```python
from build123d import *

# Parameters (mm, degrees)
F1_DEPTH  = 10
F3_D      = 2
F3_DEPTH  = 12
F3_TIP    = 0.600860619
F4_R      = 1
F5_DEPTH  = 13
F7_DEPTH  = 25
F9_DEPTH  = 9.8022701892
F11_DEPTH = 12.5


with BuildPart() as f1:
    # F0 (on Front) → F1 (new body)
    with BuildSketch(Plane.XZ):
        with BuildLine():
            Line((-4.3301270189, 21.3675134595), (-20.6698729811, -6.9337567297))
            ThreePointArc((-20.6698729811, -6.9337567297), (-20.6698729811, -11.9337567297), (-16.3397459622, -14.4337567297))
            Line((-16.3397459622, -14.4337567297), (16.3397459622, -14.4337567297))
            ThreePointArc((16.3397459622, -14.4337567297), (20.6698729811, -11.9337567297), (20.6698729811, -6.9337567297))
            Line((20.6698729811, -6.9337567297), (4.3301270189, 21.3675134595))
            ThreePointArc((4.3301270189, 21.3675134595), (0, 23.8675134595), (-4.3301270189, 21.3675134595))
        make_face()
    extrude(amount=F1_DEPTH)

    # F3
    with Locations(Plane.XZ.offset(10)):
        with Locations((0, 18.8675134595), (0, 0), (16.3397459622, -9.4337567297), (-16.3397459622, -9.4337567297)):
            Hole(F3_D / 2, depth=F3_DEPTH)
            with Locations((0, 0, -(F3_DEPTH + F3_TIP / 2))):  # 118° drill point
                Cone(0, F3_D / 2, F3_TIP, mode=Mode.SUBTRACT)

    # F4 (on face) → F5 (join)
    with BuildSketch(Plane(origin=(0, 0, 0), x_dir=(-1, 0, 0), z_dir=(0, 1, 0))):
        with BuildLine():
            Line((-7, 5.5662432703), (-7, -14.4337567297))
            Line((-7, -14.4337567297), (16.3397459622, -14.4337567297))
            ThreePointArc((16.3397459622, -14.4337567297), (20.6698729811, -11.9337567297), (20.6698729811, -6.9337567297))
            Line((20.6698729811, -6.9337567297), (4.3301270189, 21.3675134595))
            ThreePointArc((4.3301270189, 21.3675134595), (0, 23.8675134595), (-4.3301270189, 21.3675134595))
            Line((-4.3301270189, 21.3675134595), (-13.4529946162, 5.5662432703))
            Line((-13.4529946162, 5.5662432703), (-7, 5.5662432703))
        make_face()
        with Locations((16.3397459622, -9.4337567297)):
            Circle(F4_R, mode=Mode.SUBTRACT)
        Circle(F4_R, mode=Mode.SUBTRACT)
        with Locations((0, 18.8675134595)):
            Circle(F4_R, mode=Mode.SUBTRACT)
        with Locations((16.3397459622, -9.4337567297)):
            Circle(F4_R)
        Circle(F4_R)
        with Locations((0, 18.8675134595)):
            Circle(F4_R)
    extrude(amount=F5_DEPTH)

    # F6 (on face) → F7 (join)
    with BuildSketch(Plane(origin=(0, 13, 0), x_dir=(-1, 0, 0), z_dir=(0, 1, 0))):
        with BuildLine():
            Line((8.5455173281, 14.0662432703), (4.3301270189, 21.3675134595))
            ThreePointArc((4.3301270189, 21.3675134595), (0, 23.8675134595), (-4.3301270189, 21.3675134595))
            Line((-4.3301270189, 21.3675134595), (-8.5455173281, 14.0662432703))
            Line((-8.5455173281, 14.0662432703), (8.5455173281, 14.0662432703))
        make_face()
    extrude(amount=F7_DEPTH)

    # F8 (on face) → F9 (cut, through all)
    with BuildSketch(Plane(origin=(0, 0, 14.0662432703), x_dir=(1, 0, 0), z_dir=(0, 0, -1))):
        with BuildLine():
            Line((-8.5455173281, -38), (-8.5455173281, -20.0741813354))
            ThreePointArc((-8.5455173281, -20.0741813354), (-24.827324347, -44.9686543445), (4.0910069124, -38))
            Line((4.0910069124, -38), (-8.5455173281, -38))
        make_face()
        with BuildLine():
            ThreePointArc((4.0910069124, -38), (4.2102022324, -36.8778052582), (4.25, -35.75))
            ThreePointArc((4.25, -35.75), (0.6449933996, -25.6324835743), (-8.5455173281, -20.0741813354))
            Line((-8.5455173281, -20.0741813354), (-8.5455173281, -38))
            Line((-8.5455173281, -38), (4.0910069124, -38))
        make_face()
    extrude(amount=-F9_DEPTH, mode=Mode.SUBTRACT)

    # F10 (on Right) → F11 (cut, symmetric)
    with BuildSketch(Plane.YZ):
        Polygon((13, 23.8675134595), (38, 14.0662432703), (39, 14.0662432703), (39, 24.8675134595), (13, 24.8675134595), align=None)
    extrude(amount=F11_DEPTH, both=True, mode=Mode.SUBTRACT)


solid = f1.part
```
Geometry check sheet. Reference: the model listing, model coordinates, mm. A direction names the side the tool comes from. Round coordinates to 2 decimals unless told otherwise and drop trailing zeros. Write each loop counter-clockwise with the first axis right and the second up, starting at its lowest first coordinate (ties: lowest second). Pieces come first, ordered by that corner, then holes. Notation, with made-up numbers: (-33.5, 60.25) -> (-27.5, 60.25) arc R30 cw to (-27.5, 86.25) -> close; hole circle Ø10 at (59.25, 80.5). An arc over 180 degrees is marked (long way). Put each result on its own line as item: value.
1) Depth check by flat-ended pin: P1, Ø3, axis at y = -1, z = -1, coming from the +X side; P2, Ø6, axis at x = 6.5, z = -0.5, coming from the +Y side; P3, Ø6.5, axis at y = 9.5, z = -2.5, coming from the +X side. Enter the tip coordinate at first touch or a pass-through.
Recorded:
P1: stops at x = 18.11
P2: stops at y = 13
P3: stops at x = 7
2) Cross-section at D-D, the plane y = 14. Enter the section's corners in (x, z).
Recorded:
outline: (-8.55, 14.07) -> (8.55, 14.07) -> (4.33, 21.37) arc R5 ccw to (1.94, 23.48) -> (-1.94, 23.48) arc R5 ccw to (-4.33, 21.37) -> close
3) Release check for a two-part mould opening along X. For faces 1 (the face through (-17.294, -4.93, -9.133)), 2 (the face through (-20.63, 1.34, -12)), 3 (the face through (10, 6, 5.566)), 4 (the face through (-0.073, 1.219, 23.867)) record: pulls with the +X half, pulls with the -X half, needs draft (parallel to the pull), parting line crosses it, or undercut.
Recorded:
face 1: undercut
face 2: pulls with the -X half
face 3: needs draft
face 4: parting line crosses it
4) Access from +Z, -Z, +X, -X, +Y, -Y to the whole of each face (thin tool, end or side, straight path). Record for faces 5 (the face through (0, -5, -1)), 6 (the face through (12, 0, -7)), 7 (the face through (0, -10, -4)), 8 (the face through (2, 23, 14.066)).
Recorded:
face 5: -Y
face 6: -Z, +X, +Y
face 7: +Z, -Z, +X, -X, -Y
face 8: -Z, +X, -X, +Y
5) Cross-section at B-B, the plane x = 0. Enter the section's corners in (y, z).
Recorded:
outline: (-10, -14.43) -> (13, -14.43) -> (13, 14.07) -> (24.89, 14.07) -> (24.89, 19.21) -> (13, 23.87) -> (-10, 23.87) -> (-10, 19.87) -> (0, 19.87) -> (0, 17.87) -> (-10, 17.87) -> (-10, 1) -> (0, 1) -> (0, -1) -> (-10, -1) -> close
6) Cross-section at A-A, the plane y = -2. Enter the section's corners in (x, z), plus the area to 3 significant figures.
Recorded:
outline: (-20.67, -6.93) arc R5 ccw to (-16.34, -14.43) -> (16.34, -14.43) arc R5 ccw to (20.67, -6.93) -> (4.33, 21.37) arc R5 ccw to (-4.33, 21.37) -> close; hole circle Ø2 at (-16.34, -9.43); hole circle Ø2 at (0, 0); hole circle Ø2 at (0, 18.87); hole circle Ø2 at (16.34, -9.43)
area: 1,020 mm2
7) Cross-section at C-C, the plane z = 0. Enter the section's corners in (x, y).
Recorded:
outline: (-16.67, -10) -> (-1, -10) -> (-1, 0) -> (1, 0) -> (1, -10) -> (16.67, -10) -> (16.67, 0) -> (7, 0) -> (7, 13) -> (-16.67, 13) -> close
8) Thickness scan on probe 1 along Z at (x, y) = (0, -7.25); probe 2 along Y at (x, z) = (7.5, -8.5); probe 3 along Y at (x, z) = (-4, 12.5). Record the ranges inside material, lowest first. Write a range as from..to.
Recorded:
probe 1: z = -14.43..-1, 1..17.87, 19.87..23.87
probe 2: y = -10..0
probe 3: y = -10..13
